Input: part model. Units: mm. Frame: model coordinates. A direction names the side the tool comes from. Coordinates: 2 decimals unless noted, no trailing zeros. Order: outer loops, then holes, each group sorted by start corner. A loop starts at its lowest first (then second) coordinate and runs counter-clockwise, first axis right, second up.
from build123d import *

# Parameters (mm, degrees)
SKETCH2_W                        = 750
SKETCH2_H                        = 2
CUT_EXTRUDE1_START               = -75.747152873
CUT_EXTRUDE1_DEPTH               = 12.429918895
BOSS_EXTRUDE8_DEPTH              = 2
BOSS_EXTRUDE9_REACH              = 1300.889
CUT_EXTRUDE2_DEPTH               = 1250.387389222
CUT_EXTRUDE2_DEPTH_BACK          = 1250.387389222
BOSS_EXTRUDE11_REACH             = 1244.792
CUT_EXTRUDE4_DEPTH               = 1243.792388557
CUT_EXTRUDE4_DEPTH_BACK          = 1243.792388557
SKETCH9_5_W                      = 96.83734937
SKETCH9_5_H                      = 2
CUT_EXTRUDE5_DEPTH               = 1250.387389222
CUT_EXTRUDE5_DEPTH_BACK          = 1250.387389222
BOSS_EXTRUDE12_REACH             = 1251.387
BOSS_EXTRUDE12_DIRECTION_2_REACH = 1251.387
CUT_EXTRUDE6_DEPTH               = 1250.387389222


# Read off the part's stored shape, not the designer's step: Cut-Extrude1
with BuildPart() as part:
    # Sweep1: sweep along a path in Sketch1
    with BuildLine(Plane(origin=(0, 0, 0), x_dir=(0, 0, -1), z_dir=(1, 0, 0))) as sweep1_path:
        Line((412.09972218, -74.6), (622.161983643, 225.4))
        Line((622.161983643, 225.4), (794.855002782, 225.4))
        Line((794.855002782, 225.4), (794.855002782, 464.406679147))
        Line((794.855002782, 464.406679147), (873.906828676, 608.165252796))
        Line((873.906828676, 608.165252796), (873.906828676, 808.165252796))
    # Sketch2 → Sweep1 (sweep)
    with BuildSketch(Plane(origin=(0, 808.165252796, -873.906828676), x_dir=(-1, 0, 0), z_dir=(0, -1, 0))):
        with Locations((0, 1)):
            Rectangle(SKETCH2_W, SKETCH2_H)
    sweep(path=sweep1_path.line, transition=Transition.RIGHT)

    # Cut-Extrude1 outline → Cut-Extrude1 (cut)
    with BuildSketch(Plane(origin=(0, 0, 0), x_dir=(1, 0, 0), z_dir=(0, 1, 0)).offset(CUT_EXTRUDE1_START)):
        Polygon((309.004636298, 420), (250, 84.852470497), (375, 84.852470497), (375, 420), align=None)
        Polygon((-375, 84.852470497), (-250, 84.852470497), (-309.004636298, 420), (-375, 420), align=None)
    extrude(amount=CUT_EXTRUDE1_DEPTH, mode=Mode.SUBTRACT)

    # Sketch5 → Boss-Extrude8 (add)
    with BuildSketch(Plane(origin=(0, -74.6, 0), x_dir=(1, 0, 0), z_dir=(0, 1, 0))):
        Polygon((250, 84.852470497), (307.902180066, 413.738026268), (-307.902180066, 413.738026268), (-250, 84.852470497), align=None)
    extrude(amount=BOSS_EXTRUDE8_DEPTH)

    # Boss-Extrude9: up to this face of the body (flat: up to its plane)
    boss_extrude9_end = Plane(part.part.faces().sort_by_distance((0, 225.4, -708.508493212))[0])
    # Sketch7 → Boss-Extrude9 (add, up to the picked face)
    with BuildSketch(Plane(origin=(0, -74.6, 0), x_dir=(1, 0, 0), z_dir=(0, 1, 0)), mode=Mode.PRIVATE) as boss_extrude9_sk1:
        Polygon((247.969240917, 84.852470497), (250, 84.852470497), (375, 794.855002782), (372.969240917, 794.855002782), align=None)
    boss_extrude9_tool1 = split(extrude(boss_extrude9_sk1.sketch, amount=BOSS_EXTRUDE9_REACH, mode=Mode.PRIVATE), bisect_by=boss_extrude9_end, keep=Keep.BOTH, mode=Mode.PRIVATE)
    # Sketch7 → Boss-Extrude9 (add, up to the picked face)
    with BuildSketch(Plane(origin=(0, -74.6, 0), x_dir=(1, 0, 0), z_dir=(0, 1, 0)), mode=Mode.PRIVATE) as boss_extrude9_sk2:
        Polygon((-250, 84.852470497), (-247.969240917, 84.852470497), (-372.969240917, 794.855002782), (-375, 794.855002782), align=None)
    boss_extrude9_tool2 = split(extrude(boss_extrude9_sk2.sketch, amount=BOSS_EXTRUDE9_REACH, mode=Mode.PRIVATE), bisect_by=boss_extrude9_end, keep=Keep.BOTH, mode=Mode.PRIVATE)
    add(boss_extrude9_tool1.solids().sort_by(Axis((311.48462, -74.6, -439.853737), (0, 1, 0)))[0])
    add(boss_extrude9_tool2.solids().sort_by(Axis((-311.48462, -74.6, -439.853737), (0, 1, 0)))[0])

    # Sketch8 → Cut-Extrude2 (cut, two sides: drawn at the far end of the back side and taken through both)
    with BuildSketch(Plane(origin=(0, 0, 0), x_dir=(0, 0, -1), z_dir=(1, 0, 0)).offset(-CUT_EXTRUDE2_DEPTH_BACK)):
        Polygon((794.855002782, -75.747152873), (413.738026268, -75.747152873), (623.203117744, 223.4), (794.855002782, 223.4), align=None)
    extrude(amount=CUT_EXTRUDE2_DEPTH + CUT_EXTRUDE2_DEPTH_BACK, mode=Mode.SUBTRACT)

    # Boss-Extrude11: up to this plane
    boss_extrude11_end = Plane(origin=(375, 608.747952644, -874.227251213), z_dir=(0, 0.48184672916330257, 0.8762555161564617))
    # Sketch9 → Boss-Extrude11 (add, up to the surface)
    with BuildSketch(Plane(origin=(0, 808.165252796, -873.906828676), x_dir=(-1, 0, 0), z_dir=(0, -1, 0)), mode=Mode.PRIVATE) as boss_extrude11_sk1:
        Polygon((278.16265063, 0), (375, -79.051825894), (371.837349371, -79.051825894), (275, 0), align=None)
    boss_extrude11_tool1 = split(extrude(boss_extrude11_sk1.sketch, amount=BOSS_EXTRUDE11_REACH, mode=Mode.PRIVATE), bisect_by=boss_extrude11_end, keep=Keep.BOTH, mode=Mode.PRIVATE)
    add(boss_extrude11_tool1.solids().sort_by_distance((-325, 808.165253, -834.380916))[0])
    # Sketch9 → Boss-Extrude11 (add, up to the surface)
    with BuildSketch(Plane(origin=(0, 808.165252796, -873.906828676), x_dir=(-1, 0, 0), z_dir=(0, -1, 0)), mode=Mode.PRIVATE) as boss_extrude11_sk2:
        Polygon((-278.16265063, 0), (-275, 0), (-371.837349371, -79.051825894), (-375, -79.051825894), align=None)
    boss_extrude11_tool2 = split(extrude(boss_extrude11_sk2.sketch, amount=BOSS_EXTRUDE11_REACH, mode=Mode.PRIVATE), bisect_by=boss_extrude11_end, keep=Keep.BOTH, mode=Mode.PRIVATE)
    add(boss_extrude11_tool2.solids().sort_by_distance((325, 808.165253, -834.380916))[0])

    # Sketch9<5> → Cut-Extrude4 (cut, two sides: drawn at the far end of the back side and taken through both)
    with BuildSketch(Plane(origin=(0, 808.165252796, -873.906828676), x_dir=(-1, 0, 0), z_dir=(0, -1, 0)).offset(-CUT_EXTRUDE4_DEPTH_BACK)):
        with Locations((326.581325315, 1)):
            Rectangle(SKETCH9_5_W, SKETCH9_5_H)
        Polygon((375, 0), (278.16265063, 0), (375, -79.051825894), align=None)
        with Locations((-326.581325315, 1)):
            Rectangle(SKETCH9_5_W, SKETCH9_5_H)
        Polygon((-278.16265063, 0), (-375, 0), (-375, -79.051825894), align=None)
    extrude(amount=CUT_EXTRUDE4_DEPTH + CUT_EXTRUDE4_DEPTH_BACK, mode=Mode.SUBTRACT)

    # Sketch10 → Cut-Extrude5 (cut, two sides: drawn at the far end of the back side and taken through both)
    with BuildSketch(Plane(origin=(0, 0, 0), x_dir=(0, 0, -1), z_dir=(1, 0, 0)).offset(-CUT_EXTRUDE5_DEPTH_BACK)):
        Polygon((363.31001592, -74.6), (84.852470497, -2.066737554), (84.852470497, -74.6), align=None)
    extrude(amount=CUT_EXTRUDE5_DEPTH + CUT_EXTRUDE5_DEPTH_BACK, mode=Mode.SUBTRACT)

    # Boss-Extrude12: up to this face of the body (flat: up to its plane)
    boss_extrude12_end = Plane(part.part.faces().sort_by_distance((290.698054418, 99.199933477, -316.018244063))[0])
    # Sketch10<3> → Boss-Extrude12 (add, up to the picked face)
    with BuildSketch(Plane(origin=(0, 0, 0), x_dir=(0, 0, -1), z_dir=(1, 0, 0)), mode=Mode.PRIVATE) as boss_extrude12_sk1:
        Polygon((371.244288377, -74.6), (84.852470497, 0), (84.852470497, -2.066737554), (363.31001592, -74.6), align=None)
    boss_extrude12_tool1 = split(extrude(boss_extrude12_sk1.sketch, amount=BOSS_EXTRUDE12_REACH, mode=Mode.PRIVATE), bisect_by=boss_extrude12_end, keep=Keep.BOTH, mode=Mode.PRIVATE)
    add(boss_extrude12_tool1.solids().sort_by(Axis((0, -37.814265, -226.074099), (1, 0, 0)))[0])

    # Boss-Extrude12 direction 2: up to this face of the body (flat: up to its plane)
    boss_extrude12_direction_2_end = Plane(part.part.faces().sort_by_distance((-290.698054418, 99.199933477, -316.018244063))[0])
    # Sketch10<3> → Boss-Extrude12 direction 2 (add, up to the picked face)
    with BuildSketch(Plane(origin=(0, 0, 0), x_dir=(0, 0, -1), z_dir=(1, 0, 0)), mode=Mode.PRIVATE) as boss_extrude12_direction_2_sk1:
        Polygon((371.244288377, -74.6), (84.852470497, 0), (84.852470497, -2.066737554), (363.31001592, -74.6), align=None)
    boss_extrude12_direction_2_tool1 = split(extrude(boss_extrude12_direction_2_sk1.sketch, amount=-BOSS_EXTRUDE12_DIRECTION_2_REACH, mode=Mode.PRIVATE), bisect_by=boss_extrude12_direction_2_end, keep=Keep.BOTH, mode=Mode.PRIVATE)
    add(boss_extrude12_direction_2_tool1.solids().sort_by(Axis((0, -37.814265, -226.074099), (-1, 0, 0)))[0])

    # Sketch11 → Cut-Extrude6 (cut, through all)
    with BuildSketch(Plane.XY):
        with BuildLine():
            Line((-132.091535468, 997.705769529), (-362.091535468, 643.574371694))
            ThreePointArc((-362.091535468, 643.574371694), (-371.70502864, 622.723084766), (-375, 600))
            Line((-375, 600), (-375, 997.705769529))
            Line((-375, 997.705769529), (-132.091535468, 997.705769529))
        make_face()
        with BuildLine():
            Line((132.091535468, 997.705769529), (362.091535468, 643.574371694))
            ThreePointArc((362.091535468, 643.574371694), (371.70502864, 622.723084766), (375, 600))
            Line((375, 600), (375, 997.705769529))
            Line((375, 997.705769529), (132.091535468, 997.705769529))
        make_face()
    extrude(amount=-CUT_EXTRUDE6_DEPTH, mode=Mode.SUBTRACT)


solid = part.part
Item 1: Access query for faces 1 (the face through (5.206, 537.292, -834.934)), 2 (the face through (2, 225.4, -675)), 3 (the face through (-284.095, 107.425, -290.045)). Directions: +Z, -Z, +X, -X, +Y, -Y. A direction counts if a zero-diameter tool reaches every point of the face in a straight line with its end or side. Return the directions, or none.
Response values:
face 1: +Z, +Y
face 2: +Z, +X, -X, +Y
face 3: +Y
Item 2: Ray query, probe 1 along Y at (x, z) = (228, -749); probe 2 along Z at (x, y) = (58.5, 376.5) (3 decimals); probe 3 along Z at (x, y) = (-151, 608.5). Return the intervals inside material, ascending.
Response values:
probe 1: y = 223.4 to 225.4
probe 2: z = -796.855 to -794.855
probe 3: z = -875.91 to -873.91
Item 3: Cut plane C-C on z = -395. Return loops of the section in (x, y).
Response values:
outline: (-304.6, -74.6) - (304.6, -74.6) - (304.6, 225.4) - (302.57, 225.4) - (302.57, -72.6) - (-302.57, -72.6) - (-302.57, 225.4) - (-304.6, 225.4) - close
Item 4: Cut plane B-B on y = 25. Return loops of the section in (x, z), then the cut area to 3 significant figures.
Response values:
outline: (-375, -484.28) - (375, -484.28) - (375, -481.84) - (319.89, -481.84) - (250, -84.85) - (247.97, -84.85) - (317.86, -481.84) - (-317.86, -481.84) - (-247.97, -84.85) - (-250, -84.85) - (-319.89, -481.84) - (-375, -481.84) - close
area: 3,440 mm2
Item 5: Draft query along X for faces 4 (the face through (4, 710, -873.907)), 5 (the face through (-4, 709, -875.907)), 6 (the face through (-326.355, 601.123, -834.565)). Return one class per face: pulls with the +X half, pulls with the -X half, needs draft (parallel to the pull), parting line crosses it, or undercut.
Response values:
face 4: undercut
face 5: needs draft
face 6: pulls with the -X half
Item 6: Cut plane A-A on x = -78. Return loops of the section in (y, z) (3 decimals).
Response values:
outline: (-75.747, -413.738) - (223.4, -623.203) - (223.4, -796.855) - (463.893, -796.855) - (607.652, -875.907) - (808.165, -875.907) - (808.165, -873.907) - (608.165, -873.907) - (464.407, -794.855) - (225.4, -794.855) - (225.4, -622.162) - (-72.6, -413.5) - (-72.6, -363.566) - (0, -84.852) - (-2.067, -84.852) - (-74.6, -363.31) - (-74.6, -412.1) - close
Item 7: Pin query (flat end, axial travel): pin 1 Ø2 at (x, z) = (204, -290.5) entering from +Y; pin 2 Ø12 at (x, y) = (73, 565) entering from +Z; pin 3 Ø0.6 at (y, z) = (669.5, -875.5) entering from +X. Return the tip coordinate at first contact, or that it passes through.
Response values:
pin 1: stops at y = -53.31
pin 2: stops at z = -846.87
pin 3: stops at x = 278.16
Item 8: Cut plane D-D on y = 663. Return loops of the section in (x, z).
Response values:
outline: (-349.48, -815.69) - (-278.16, -873.91) - (-278.16, -875.91) - (278.16, -875.91) - (278.16, -873.91) - (349.48, -815.69) - (349.48, -813.11) - (275, -873.91) - (-275, -873.91) - (-349.48, -813.11) - close
